from build123d import *

# Parameters (mm, degrees)
SKETCH_1_W           = 60
SKETCH_1_H           = 34
EXTRUDE_1_DEPTH      = 20
CUT_EXTRUDE_8_DEPTH  = 66
SKETCH_20_W          = 5
SKETCH_20_H          = 34
EXTRUDE_7_DEPTH      = 20
SKETCH_22_W          = 65
SKETCH_22_H          = 20
EXTRUDE_8_DEPTH      = 7
SKETCH_21_R          = 1.5
CUT_EXTRUDE_13_DEPTH = 58.497826046
CUT_EXTRUDE_START    = -41
SKETCH_23_W          = 65
SKETCH_23_H          = 20
CUT_EXTRUDE_14_DEPTH = 17
CUT_EXTRUDE_16_DEPTH = 4.2
SKETCH_27_W          = 8
SKETCH_27_H          = 12
EXTRUDE_10_DEPTH     = 14
SKETCH_30_R          = 1.5
CUT_EXTRUDE_18_DEPTH = 54.150729064
FILLET_6_R           = 5
CUT_EXTRUDE_22_DEPTH = 5
SKETCH_36_R          = 1.35
CUT_EXTRUDE_23_DEPTH = 54.150729064


with BuildPart() as part:
    # 草图1 → 凸台-拉伸1 (new body)
    with BuildSketch(Plane.XY):
        Rectangle(SKETCH_1_W, SKETCH_1_H)
    extrude(amount=EXTRUDE_1_DEPTH)

    # 草图19 → 切除-拉伸8 (cut)
    with BuildSketch(Plane.XY.offset(20)):
        with BuildLine():
            Line((0, 9), (-1, 9))
            ThreePointArc((-1, 9), (-10, 0), (-1, -9))
            Line((-1, -9), (0.07899986, -9))
            Line((0.07899986, -9), (9.502211487, -5.541477859))
            ThreePointArc((9.502211487, -5.541477859), (11, 0), (9.502211487, 5.541477859))
            Line((9.502211487, 5.541477859), (0, 9))
        make_face()
    extrude(amount=-CUT_EXTRUDE_8_DEPTH, mode=Mode.SUBTRACT)

    # 草图20 → 凸台-拉伸7 (add)
    with BuildSketch(Plane.XY.offset(20)):
        with Locations((-32.5, 0)):
            Rectangle(SKETCH_20_W, SKETCH_20_H)
    extrude(amount=-EXTRUDE_7_DEPTH)

    # 草图22 → 凸台-拉伸8 (add)
    with BuildSketch(Plane.XZ.offset(17)):
        with Locations((-2.5, 10)):
            Rectangle(SKETCH_22_W, SKETCH_22_H)
    extrude(amount=EXTRUDE_8_DEPTH)

    # 草图21 → 切除-拉伸13 (cut, through all)
    with BuildSketch(Plane.XZ.offset(-17)):
        with Locations(Location((-28.5, 10, 0), (0, 0, 90))):
            Circle(SKETCH_21_R)
        with Locations(Location((23.5, 10, 0), (0, 0, 270))):
            Circle(SKETCH_21_R)
    extrude(amount=CUT_EXTRUDE_13_DEPTH, mode=Mode.SUBTRACT)

    # 草图23 → 切除-拉伸14 (cut)
    with BuildSketch(Plane.XZ.offset(24).offset(CUT_EXTRUDE_START)):
        with Locations((-2.5, 10)):
            Rectangle(SKETCH_23_W, SKETCH_23_H)
    extrude(amount=CUT_EXTRUDE_14_DEPTH, mode=Mode.SUBTRACT)

    # 草图25 → 切除-拉伸16 (cut)
    with BuildSketch(Plane(origin=(0, 0, 0), x_dir=(1, 0, 0), z_dir=(0, 1, 0))):
        Polygon((26.733161507, -10), (25.116580754, -7.2), (21.883419246, -7.2), (20.266838493, -10), (21.883419246, -12.8), (25.116580754, -12.8), align=None)
        Polygon((-25.266838493, -10), (-26.883419246, -7.2), (-30.116580754, -7.2), (-31.733161507, -10), (-30.116580754, -12.8), (-26.883419246, -12.8), align=None)
    extrude(amount=-CUT_EXTRUDE_16_DEPTH, mode=Mode.SUBTRACT)

    # 草图27 → 凸台-拉伸10 (add)
    with BuildSketch(Plane(origin=(0, 0, 0), x_dir=(1, 0, 0), z_dir=(0, 1, 0))):
        with Locations((34, -10)):
            Rectangle(SKETCH_27_W, SKETCH_27_H)
        with Locations((-39, -10)):
            Rectangle(SKETCH_27_W, SKETCH_27_H)
    extrude(amount=-EXTRUDE_10_DEPTH)

    # 草图30 → 切除-拉伸18 (cut, through all)
    with BuildSketch(Plane(origin=(0, 0, 0), x_dir=(1, 0, 0), z_dir=(0, 1, 0))):
        with Locations(Location((34, -10, 0), (0, 0, 270))):
            Circle(SKETCH_30_R)
        with Locations(Location((-39, -10, 0), (0, 0, 270))):
            Circle(SKETCH_30_R)
    extrude(amount=-CUT_EXTRUDE_18_DEPTH, mode=Mode.SUBTRACT)

    # 圆角6
    # the kernel refuses this fillet: 5 mm, written as the material it adds along each edge
    with BuildSketch(Plane(origin=(-35, 0, 4), x_dir=(-1.5685230891899147e-12, 0, -1.0), z_dir=(0, -1, 0)), Plane(origin=(30, 0, 16), x_dir=(1.5978329770400045e-12, 0, 1.0), z_dir=(0, -1, 0))) as fillet_6_piece_1:
        with BuildLine():
            CenterArc((5, -4.898979486), FILLET_6_R, 101.536959033, 78.463040967)
            Line((0, -4.898979486), (-0.1, -4.898979486))
            Line((-0.1, -4.898979486), (-0.1, 0))
            Line((-0.1, 0), (0, 0.1))
            ThreePointArc((0, 0.1), (2, 0.1), (3.98, 0.09797959))
            Line((3.98, 0.09797959), (4, 0))
        make_face()
    extrude(amount=14)
    with BuildSketch(Plane(origin=(-35, 0, 16), x_dir=(-1.596944798620306e-12, 0, 1.0), z_dir=(0, -1, 0)), Plane(origin=(30, 0, 4), x_dir=(1.5702994460293186e-12, 0, -1.0), z_dir=(0, -1, 0))) as fillet_6_piece_2:
        with BuildLine():
            CenterArc((5, 4.898979486), FILLET_6_R, 180, 78.463040967)
            Line((0, 4.898979486), (-0.1, 4.898979486))
            Line((-0.1, 4.898979486), (-0.1, 0))
            Line((-0.1, 0), (0, -0.1))
            ThreePointArc((0, -0.1), (2, -0.1), (3.98, -0.09797959))
            Line((3.98, -0.09797959), (4, 0))
        make_face()
    extrude(amount=14)

    # 草图35 → 切除-拉伸22 (cut)
    with BuildSketch(Plane.XZ.offset(14)):
        Polygon((37.117691454, 10), (35.558845727, 12.7), (32.441154273, 12.7), (30.882308546, 10), (32.441154273, 7.3), (35.558845727, 7.3), align=None)
        Polygon((-35.882308546, 10), (-37.441154273, 12.7), (-40.558845727, 12.7), (-42.117691454, 10), (-40.558845727, 7.3), (-37.441154273, 7.3), align=None)
    extrude(amount=-CUT_EXTRUDE_22_DEPTH, mode=Mode.SUBTRACT)

    # 草图36 → 切除-拉伸23 (cut, through all)
    with BuildSketch(Plane.XZ.offset(24)):
        with Locations(Location((0, 15, 0), (0, 0, 270))):
            Circle(SKETCH_36_R)
    extrude(amount=-CUT_EXTRUDE_23_DEPTH, mode=Mode.SUBTRACT)


solid = part.part
Geometry check sheet. Reference: the model listing, model coordinates, mm. A direction names the side the tool comes from. Give positions to 0.01 mm unless a question says otherwise; leave off trailing zeros. Order: outer loops, then holes, each group sorted by start corner. A loop starts at its lowest first (then second) coordinate and runs counter-clockwise, first axis right, second up.
1) Draft check along X on faces 5 (the flat face through (30, -19, 10)), 6 (the flat face through (34, -12, 7.3)), 7 (the flat face through (-3, -12, 0)). Enter one of: released by +X, released by -X, zero draft, split by the parting line, or undercut.
Results are:
face 5: released by +X
face 6: undercut
face 7: zero draft
2) Material ranges on probe 1 along X at (y, z) = (-20.5, 10); probe 2 along X at (y, z) = (-9.5, 10); probe 3 along X at (y, z) = (-16.5, 15), recorded low to high.
Results are:
probe 1: x = -35 to -30, -27 to 22, 25 to 30
probe 2: x = -43 to -42.12, -35.88 to -30, -27 to 22, 25 to 30.88, 37.12 to 38
probe 3: x = -35 to -1.35, 1.35 to 30
3) Cross-section at A-A (x = -28.5). Record the boundary of the cut face in (y, z), then the cut area to 3 significant figures.
Results are:
outline: (-24, 0) - (0, 0) - (0, 7.2) - (-4.2, 7.2) - (-4.2, 8.5) - (-24, 8.5) - close; (-24, 11.5) - (-4.2, 11.5) - (-4.2, 12.8) - (0, 12.8) - (0, 20) - (-24, 20) - close
area: 397 mm2
4) Gauge pin test, flat ends, axial feed: pin 1 (6.5 mm diameter, centred on x = 34, z = 7, fed in from -Y); pin 2 (3.5 mm diameter, centred on x = -38.5, y = -11, fed in from -Z); pin 3 (0.9 mm diameter, centred on x = -0.5, z = 18.5, fed in from +Y). Record the tip position at first contact, or that the pin passes through.
Results are:
pin 1: stops at y = -14
pin 2: stops at z = 2.88
pin 3: stops at y = -9
5) Tool access check on faces 1 (the flat face through (-41, -7, 4)), 2 (the flat face through (-36.673, -11.535, 8.631)), 3 (the cylindrical face through (-7.434, -6.294, 10.14)), 4 (the flat face through (24, -2, 7.2)). Record the directions out of +Z, -Z, +X, -X, +Y, -Y that give a thin tool (end or side, any length) a straight path to the whole face; none if there is none.
Results are:
face 1: -Z, -X, +Y, -Y
face 2: -Y
face 3: +Z, -Z, +Y
face 4: +Y
6) Cross-section at D-D (z = 15). Record the boundary of the cut face in (x, y).
Results are:
outline: (-43, -14) - (-35, -14) - (-35, -24) - (-1.35, -24) - (-1.35, -8.99) arc R9 cw to (-10, 0) - (-43, 0) - close; (1.35, -24) - (30, -24) - (30, -14) - (38, -14) - (38, 0) - (11, 0) arc R11 cw to (9.5, -5.54) - (1.35, -8.53) - close
7) Cross-section at C-C (y = -13.25). Record the boundary of the cut face in (x, z), then the cut area to 3 significant figures.
Results are:
outline: (-43, 4) - (-39.9, 4) arc R5 cw to (-35, 0) - (30, 0) arc R5 cw to (34.9, 4) - (38, 4) - (38, 16) - (34.9, 16) arc R5 cw to (30, 20) - (-35, 20) arc R5 cw to (-39.9, 16) - (-43, 16) - close; hole (-42.12, 10) - (-40.56, 7.3) - (-37.44, 7.3) - (-35.88, 10) - (-37.44, 12.7) - (-40.56, 12.7) - close; hole circle Ø3 at (-28.5, 10); hole circle Ø2.7 at (0, 15); hole circle Ø3 at (23.5, 10); hole (30.88, 10) - (32.44, 7.3) - (35.56, 7.3) - (37.12, 10) - (35.56, 12.7) - (32.44, 12.7) - close
area: 1,440 mm2
8) Cross-section at B-B (y = -18). Record the boundary of the cut face in (x, z), then the cut area to 3 significant figures.
Results are:
outline: (-35, 0) - (30, 0) - (30, 20) - (-35, 20) - close; hole circle Ø3 at (-28.5, 10); hole circle Ø2.7 at (0, 15); hole circle Ø3 at (23.5, 10)
area: 1,280 mm2
